Could you check a few things on this model? Use its own coordinates, in mm. Coordinates: 2 decimals unless noted, no trailing zeros. Order: outer loops, then holes, each group sorted by start corner. A loop starts at its lowest first (then second) coordinate and runs counter-clockwise, first axis right, second up. Notation, with made-up numbers: (57, 71) -> (64, 71) arc R12 ccw to (64, 93) -> close; hole circle Ø2 at (-10, 38.5). An arc over 180 degrees is marked (long way). Use a Markdown table: item, result. Add a question column.
1) If I drill on L1, parallel to X at y = 12, z = 22; L2, parallel to X at y = 8.5, z = 26.5, over which ranges is the centre line in solid material (lowest first)? Write a range as [from, to].
2) If we section it at B-B (z = 28): Write out the boundary of the cut face in (x, y).
3) If we section it at D-D (x = 212): Write out the boundary of the cut face in (y, z).
4) If we section it at A-A (y = 3.5): Write out the boundary of the cut face in (x, z), plus the area to 3 significant figures.
5) If we section it at C-C (x = 24): Write out the boundary of the cut face in (y, z), plus the area to 3 significant figures.
6) Thinking about a two-plate mould opening in X: for faces 1 (the flat face through (118, 8, 0)), 2 (the flat face through (240, 7, 22)), 3 (the cylindrical face through (18.95, 7.605, 15.413)), which applies, +X half, -X half, draft (parallel to the pull), parting line (faces both ways), or undercut?
```python
from build123d import *

# Parameters (mm, degrees)
SKETCH_1_W          = 240
SKETCH_1_H          = 15
TOP_BEAM_DEPTH      = 44
SKETCH_2_R          = 8.3
SCREW_PASSAGE_DEPTH = 245.460630777
SKETCH_3_R          = 8.3
CUT_EXTRUDE_2_DEPTH = 245.460630777


with BuildPart() as part:
    # 草图1 → Top_beam (new body)
    with BuildSketch(Plane.XY):
        with Locations((120, 7.5)):
            Rectangle(SKETCH_1_W, SKETCH_1_H)
    extrude(amount=TOP_BEAM_DEPTH)

    # 草图2 → Screw_passage (cut, through all)
    with BuildSketch(Plane(origin=(0, 15, 0), x_dir=(1, 0, 0), z_dir=(0, 1, 0))):
        with Locations(Location((24, -22, 0), (0, 0, 270))):
            Circle(SKETCH_2_R)
    extrude(amount=-SCREW_PASSAGE_DEPTH, mode=Mode.SUBTRACT)

    # 草图3 → 切除-拉伸2 (cut, through all)
    with BuildSketch(Plane(origin=(0, 15, 0), x_dir=(1, 0, 0), z_dir=(0, 1, 0))):
        with Locations(Location((216, -22, 0), (0, 0, 270))):
            Circle(SKETCH_3_R)
    extrude(amount=-CUT_EXTRUDE_2_DEPTH, mode=Mode.SUBTRACT)


solid = part.part
```
Answer sheet:
| question | item | result |
|---|---|---|
| 1 | L1 | [0, 15.7], [32.3, 207.7], [224.3, 240] |
| 1 | L2 | [0, 17.03], [30.97, 209.03], [222.97, 240] |
| 2 | outline | (0, 0) -> (18.27, 0) -> (18.27, 15) -> (0, 15) -> close; (29.73, 0) -> (210.27, 0) -> (210.27, 15) -> (29.73, 15) -> close; (221.73, 0) -> (240, 0) -> (240, 15) -> (221.73, 15) -> close |
| 3 | outline | (0, 0) -> (15, 0) -> (15, 14.73) -> (0, 14.73) -> close; (0, 29.27) -> (15, 29.27) -> (15, 44) -> (0, 44) -> close |
| 4 | outline | (0, 0) -> (240, 0) -> (240, 44) -> (0, 44) -> close; hole circle Ø16.6 at (24, 22); hole circle Ø16.6 at (216, 22) |
| 4 | area | 10,100 mm2 |
| 5 | outline | (0, 0) -> (15, 0) -> (15, 13.7) -> (0, 13.7) -> close; (0, 30.3) -> (15, 30.3) -> (15, 44) -> (0, 44) -> close |
| 5 | area | 411 mm2 |
| 6 | face 1 | draft |
| 6 | face 2 | +X half |
| 6 | face 3 | undercut |
